Autodesk Inventor part; units mm, degrees
ref_plane "YZ Plane" through (0, 0, 0) normal (1, 0, 0) x (0, 1, 0)
ref_plane "XZ Plane" through (0, 0, 0) normal (0, 1, 0) x (-1, 0, 0)
ref_plane "XY Plane" through (0, 0, 0) normal (0, 0, 1) x (1, 0, 0)
sketch "Sketch1" plane through (0, 0, 0) normal (0, 0, 1) x (1, 0, 0)
  line L0 (-16.2709, 3) -> (-16.2709, 0)
  line L1 (-33.7709, 3) -> (-16.2709, 3)
  line L2 (-33.7709, 0) -> (-33.7709, 3)
  line L3 (-33.7709, 0) -> (-48.7992, 0)
  line L4 (-30.0209, 63) -> (-20.0209, 63)
  line L5 (-20.0209, 63) -> (-20.0209, 60)
  line L6 (-30.0209, 60) -> (-30.0209, 63)
  line L7 (-30.0209, 63) -> (-20.0209, 60) construction
  line L8 (-20.0209, 63) -> (-30.0209, 60) construction
  line L9 (-25.4776, 30) -> (-35.4566, 30) construction
  line L10 (-25.0209, 30) -> (-25.0209, 38) construction
  line L11 (-45.0209, 63) -> (-35.0209, 63)
  line L12 (-35.0209, 63) -> (-35.0209, 60)
  line L13 (-45.0209, 60) -> (-45.0209, 63)
  line L14 (-45.0209, 63) -> (-35.0209, 60) construction
  line L15 (-35.0209, 63) -> (-45.0209, 60) construction
  line L16 (-15.0209, 63) -> (-5.0209, 63)
  line L17 (-5.0209, 63) -> (-5.0209, 60)
  line L18 (-15.0209, 60) -> (-15.0209, 63)
  line L19 (-15.0209, 63) -> (-5.0209, 60) construction
  line L20 (-5.0209, 63) -> (-15.0209, 60) construction
  line L21 (-30.0209, 63) -> (-20.0209, 63)
  line L22 (-20.0209, 63) -> (-20.0209, 60)
  line L23 (-30.0209, 60) -> (-30.0209, 63)
  line L24 (-30.0209, 63) -> (-20.0209, 60) construction
  line L25 (-20.0209, 63) -> (-30.0209, 60) construction
  line L26 (-48.7992, 60) -> (-45.0209, 60)
  line L27 (-35.0209, 60) -> (-30.0209, 60)
  line L28 (-20.0209, 60) -> (-15.0209, 60)
  line L29 (-48.7992, 15) -> (-51.799, 15)
  line L30 (-51.799, 15) -> (-51.799, 25)
  line L31 (-51.799, 25) -> (-48.7992, 25)
  line L32 (-48.7992, 35) -> (-51.799, 35)
  line L33 (-51.799, 35) -> (-51.799, 45)
  line L34 (-48.7992, 45) -> (-51.799, 45)
  line L35 (-48.7992, 55) -> (-51.7992, 55)
  line L36 (-48.7992, 55) -> (-45.7992, 55) construction
  line L37 (-51.7992, 55) -> (-51.7992, 60)
  line L38 (-51.7992, 60) -> (-48.7992, 60)
  line L39 (-48.7992, 55) -> (-48.7992, 45)
  line L40 (-48.7992, 35) -> (-48.7992, 25)
  line L41 (-48.7992, 15) -> (-48.7992, 5)
  line L42 (-48.7992, 5) -> (-51.7992, 5)
  line L43 (-51.7992, 5) -> (-51.7992, 0)
  line L44 (-51.7992, 0) -> (-48.7992, 0)
  line L45 (-16.2709, 0) -> (-1.2426, 0)
  line L46 (-1.2426, 60) -> (-5.0209, 60)
  line L47 (-1.2426, 15) -> (1.7572, 15)
  line L48 (1.7572, 15) -> (1.7572, 25)
  line L49 (1.7572, 25) -> (-1.2426, 25)
  line L50 (-1.2426, 35) -> (1.7572, 35)
  line L51 (1.7572, 35) -> (1.7572, 45)
  line L52 (-1.2426, 45) -> (1.7572, 45)
  line L53 (-1.2426, 55) -> (1.7574, 55)
  line L54 (1.7574, 55) -> (1.7574, 60)
  line L55 (1.7574, 60) -> (-1.2426, 60)
  line L56 (-1.2426, 55) -> (-1.2426, 45)
  line L57 (-1.2426, 35) -> (-1.2426, 25)
  line L58 (-1.2426, 15) -> (-1.2426, 5)
  line L59 (-1.2426, 5) -> (1.7574, 5)
  line L60 (1.7574, 5) -> (1.7574, 0)
  line L61 (1.7574, 0) -> (-1.2426, 0)
  circle A0 centre (-44.3959, 23.1933) radius 1.5875
  circle A1 centre (-44.3959, 7.0713) radius 1.5875
  circle A2 centre (-36.7209, 15.1323) radius 8.25
  circle A3 centre (-25.0211, 22.0323) radius 2.95
  circle A4 centre (-25.0211, 8.2323) radius 2.95
  circle A5 centre (-13.3209, 15.1323) radius 8.25
  circle A6 centre (-5.6459, 7.0713) radius 1.5875
  circle A7 centre (-5.6459, 23.1933) radius 1.5875
  circle A8 centre (-41.9566, 29.25) radius 1.5
  circle A9 centre (-41.5, 48) radius 1.5
  line L62 (-5.6459, 7.0713) -> (-44.3959, 23.1933) construction
  line L63 (-44.3959, 23.1933) -> (-5.6459, 23.1933) construction
  line L64 (-5.6459, 23.1933) -> (-44.3959, 7.0713) construction
  point P0 (0, 0)
  point P1 (-25.0209, 61.5)
  point P2 (-40.0209, 61.5)
  point P3 (-10.0209, 61.5)
  point P4 (-25.0209, 61.5)
  point P5 (-48.7992, 30)
  point P6 (-1.2426, 30)
  point P7 (-25.4776, 15.3162)
  point P8 (-25.4776, 15.3162)
  point P9 (-25.4776, 15.3162)
  point P10 (-25.4776, 15.3162)
  point P11 (-25.0209, 3)
  point P12 (-25.0209, 15.1323)
  dimension "d0" = 10
  dimension "d1" = 3
  dimension "d4" = 15
  dimension "d7" = 15
  dimension "d13" = 3
  dimension "d14" = 180
  dimension "d15" = 3
  dimension "d17" = 7.675
  dimension "d18" = 7.675
  dimension "d23" = 2.9998
  dimension "d30" = 11.7002
  dimension "d31" = 11.6998
  dimension "d32" = 7.675
  dimension "d33" = 7.675
  dimension "d34" = 11.6998
  dimension "d35" = 11.7002
  dimension "d45" = 8.061
  dimension "d46" = 8.061
extrude "Extrusion2" add sketch "Sketch1" along normal blind 3
sketch "Sketch2" plane through (0, 0, 3) normal (0, 0, 1) x (1, 0, 0)
  line L0 (-1.2426, 5) -> (-1.2426, 15)
  line L1 (-1.2426, 25) -> (-1.2426, 35)
  line L2 (-1.2426, 45) -> (-1.2426, 55)
  line L3 (-48.7992, 55) -> (-48.7992, 45)
  line L4 (-48.7992, 35) -> (-48.7992, 25)
  line L5 (-48.7992, 15) -> (-48.7992, 5)
  line L6 (-1.2426, 5) -> (-2.2426, 5)
  line L7 (-2.2426, 5) -> (-2.2426, 15)
  line L8 (-2.2426, 15) -> (-1.2426, 15)
  line L9 (-1.2426, 25) -> (-2.2426, 25)
  line L10 (-2.2426, 25) -> (-2.2426, 35)
  line L11 (-2.2426, 35) -> (-1.2426, 35)
  line L12 (-1.2426, 45) -> (-2.2426, 45)
  line L13 (-2.2426, 45) -> (-2.2426, 55)
  line L14 (-2.2426, 55) -> (-1.2426, 55)
  line L15 (-48.7992, 5) -> (-47.7992, 5)
  line L16 (-47.7992, 5) -> (-47.7992, 15)
  line L17 (-47.7992, 15) -> (-48.7992, 15)
  line L18 (-48.7992, 25) -> (-47.7992, 25)
  line L19 (-47.7992, 25) -> (-47.7992, 35)
  line L20 (-47.7992, 35) -> (-48.7992, 35)
  line L21 (-48.7992, 45) -> (-47.7992, 45)
  line L22 (-48.7992, 45) -> (-51.799, 45)
  line L23 (-47.7992, 45) -> (-47.7992, 55)
  line L24 (-47.7992, 55) -> (-48.7992, 55)
  point P0 (0, 0)
  dimension "d24" = 1
  dimension "d25" = 1
  dimension "d28" = 1
  dimension "d29" = 1
extrude "Extrusion3" cut sketch "Sketch2" against normal through all
sketch "Sketch3" plane through (0, 0, 3) normal (0, 0, 1) x (1, 0, 0)
  line L0 (1.7574, 60) -> (-5.0209, 60)
  line L1 (1.7574, 0) -> (-0.2426, 0)
  line L2 (-0.2426, 0) -> (-0.2426, 60)
  line L3 (-0.2426, 60) -> (1.7574, 60)
  line L4 (1.7574, 60) -> (1.7574, 0)
  line L5 (-45.0209, 60) -> (-51.7992, 60)
  line L6 (-51.7992, 0) -> (-49.7992, 0)
  line L7 (-49.7992, 0) -> (-49.7992, 60)
  line L8 (-49.7992, 60) -> (-51.7992, 60)
  line L9 (-51.7992, 60) -> (-51.7992, 0)
  point P0 (0, 0)
  dimension "d47" = 2
  dimension "d48" = 2
extrude "Extrusion4" cut sketch "Sketch3" against normal through all
sketch "Sketch4" plane through (0, 0, 3) normal (0, 0, 1) x (1, 0, 0)
  line L0 (-2.2426, 5) -> (-0.2426, 5)
  line L1 (-0.2426, 5) -> (-0.2426, 0)
  line L2 (-0.2426, 0) -> (-2.2426, 0)
  line L3 (-2.2426, 0) -> (-2.2426, 5)
  line L4 (-47.7992, 5) -> (-49.7992, 5)
  line L5 (-49.7992, 5) -> (-49.7992, 0)
  line L6 (-49.7992, 0) -> (-47.7992, 0)
  line L7 (-47.7992, 0) -> (-47.7992, 5)
  point P0 (0, 0)
extrude "Extrusion5" cut sketch "Sketch4" against normal through all
equation "\"d46\" = d45"
equation "\"d25\" = d24"
equation "\"d28\" = d24"
equation "\"d29\" = d24"
equation "\"d48\" = d47"
properties part number "srf diag kanan"
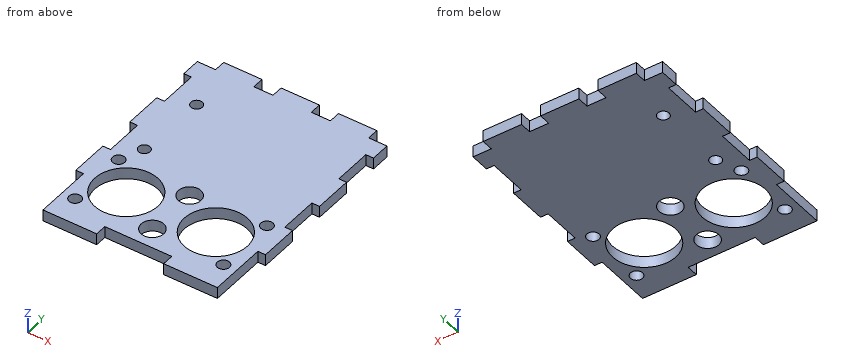
The model under review builds one solid part; all positions refer to its coordinate system, in mm. Round coordinates to 2 decimals unless told otherwise and drop trailing zeros. Loops run counter-clockwise (first coordinate to the right, second up) from the corner with the lowest first, then second, coordinate; pieces in that order, holes last. Notation, with made-up numbers: (-12.5, 28) -> (0.5, 28) arc R24 cw to (0.5, 57) -> close; hole circle Ø9 at (11.25, 75.5). An arc over 180 degrees is marked (long way). One line per question, with ' | ' between items. Start each with the question number.
Item 1: Add section A-A, the plane x = -41.5. Write out the cut boundary in (y, z).
Item 2: Add section B-B, the plane y = 29.25. Write out the cut boundary in (x, z), then the cut area to 3 significant figures.
Item 3: Add section D-D, the plane x = -31.5. Write out the cut boundary in (y, z).
Item 4: Wall thickness on line 1 along X through (y, z) = (9.5, 0.85); line 2 along X through (y, z) = (6.5, 0.25); line 3 along X through (y, z) = (22, 1.2): over which ranges is each line inside the solid? List them lowest first. Write a range as [from, to].
Item 5: For pin 1 (0.6 mm diameter, centred on x = -48.5, z = 1.5, fed in from -Y); pin 2 (1.6 mm diameter, centred on x = -1.5, z = 1.5, fed in from +Y); pin 3 (1.5 mm diameter, centred on y = 61, z = 2, fed in from +X), all flat-tipped, find the tip position at first contact; note any pin that passes through.
Item 6: Add section C-C, the plane y = 16. Write out the cut boundary in (x, z).
Return value:
1) outline: (0, 0) -> (8.41, 0) -> (8.41, 3) -> (0, 3) -> close; (21.86, 0) -> (27.82, 0) -> (27.82, 3) -> (21.86, 3) -> close; (30.68, 0) -> (46.5, 0) -> (46.5, 3) -> (30.68, 3) -> close; (49.5, 0) -> (63, 0) -> (63, 3) -> (49.5, 3) -> close
2) outline: (-47.8, 0) -> (-43.46, 0) -> (-43.46, 3) -> (-47.8, 3) -> close; (-40.46, 0) -> (-2.24, 0) -> (-2.24, 3) -> (-40.46, 3) -> close | area: 128 mm2
3) outline: (3, 0) -> (8.74, 0) -> (8.74, 3) -> (3, 3) -> close; (21.52, 0) -> (60, 0) -> (60, 3) -> (21.52, 3) -> close
4) line 1: x = [-47.8, -42.75], [-30.69, -27.68], [-22.36, -19.35], [-7.29, -2.24] | line 2: x = [-47.8, -45.88], [-42.91, -27.41], [-22.63, -7.13], [-4.16, -2.24] | line 3: x = [-49.8, -45.44], [-43.35, -41.29], [-32.15, -27.97], [-22.07, -17.89], [-8.75, -6.69], [-4.6, -0.24]
5) pin 1: stops at y = 15 | pin 2: stops at y = 60 | pin 3: stops at x = -5.02
6) outline: (-49.8, 0) -> (-44.93, 0) -> (-44.93, 3) -> (-49.8, 3) -> close; (-28.52, 0) -> (-21.53, 0) -> (-21.53, 3) -> (-28.52, 3) -> close; (-5.12, 0) -> (-0.24, 0) -> (-0.24, 3) -> (-5.12, 3) -> close
